```python
from build123d import *

# Parameters (mm, degrees)
F0_W        = 457.2
F0_H        = 88.9
F1_DEPTH    = 12.7
F3_DEPTH    = 12.701
F4_T1_DEPTH = 425.4697854373
F4_T3_DEPTH = 32.2962243683
F4_T5_DEPTH = 24.3646579033


# Not quite as in the source:
# - a fillet or chamfer that OpenCascade refuses, or shapes differently, is made with other operations: its cross-section is extruded or revolved along the edge and cut away or added
# - a feature names something its author has since deleted; it is built from what else it names


with BuildPart() as f1:
    # F0 (on Front) → F1 (new body)
    with BuildSketch(Plane.XZ):
        Rectangle(F0_W, F0_H)
    extrude(amount=F1_DEPTH)

    # F2 (on face) → F3 (cut, through all)
    with BuildSketch(Plane.XZ.offset(12.7)):
        Polygon((-177.273561069, -44.45), (-228.6, 44.45), (-228.6, -44.45), align=None)
    extrude(amount=-F3_DEPTH, mode=Mode.SUBTRACT)

    # F4: chamfer of 3.81 on 4 edges, made by hand

    # F4_s2 → F4_t1 (cut)
    with BuildSketch(Plane.YZ.offset(-187.0716732532)):
        Polygon((0, -40.64), (-3.81, -44.45), (0, -44.45), align=None)
        Polygon((-12.7, -40.64), (-8.89, -44.45), (-12.7, -44.45), align=None)
    extrude(amount=F4_T1_DEPTH, mode=Mode.SUBTRACT)

    # F4_s4 → F4_t3 (cut)
    with BuildSketch(Plane.XZ.offset(-9.7981121842)):
        Polygon((228.6, -40.64), (224.79, -44.45), (228.6, -44.45), align=None)
    extrude(amount=F4_T3_DEPTH, mode=Mode.SUBTRACT)

    # F4_s6 → F4_t5 (cut)
    with BuildSketch(Plane.XZ.offset(-5.8323289516)):
        Polygon((-178.3734133318, -42.545), (-175.0738565434, -44.45), (-177.273561069, -44.45), align=None)
    extrude(amount=F4_T5_DEPTH, mode=Mode.SUBTRACT)


solid = f1.part
```
The listing builds one solid part. Answer for the finished solid, in the listing's coordinates (mm). Round coordinates to 2 decimals unless told otherwise and drop trailing zeros. Order: outer loops, then holes, each group sorted by start corner. A loop starts at its lowest first (then second) coordinate and runs counter-clockwise, first axis right, second up. Notation, with made-up numbers: (-15, 18.25) - (5, 18.25) arc R11 ccw to (5, 37.25) - close; hole circle Ø10 at (6, 1.5). An arc over 180 degrees is marked (long way). Put each result on its own line as item: value. Start each with the question number.
(1) Straight lines are drawn through the part: probe 1 along Z at (x, y) = (-54.5, -12); probe 2 along Z at (x, y) = (127.5, -1); probe 3 along X at (y, z) = (-4, -1). For each, find the intervals that lie inside material, in ascending order. Write a range as from..to.
(2) Given P1, Ø5, axis at y = -3, z = 12, coming from the -X side; P2, Ø1, axis at x = -43, y = -10, coming from the -Z side, each flat-ended and moving along its own axis, determine where each tip first touches the part or whether it passes through.
(3) Find section C-C (z = 21.5). Give the vertices of the cut face in (x, y), plus the area to 3 significant figures.
(4) Find section A-A (y = -6). Give the vertices of the cut face in (x, z) (3 decimals).
(5) Find section B-B (z = -13.5). Give the vertices of the cut face in (x, y), plus the area to 3 significant figures.
Reply:
1. probe 1: -41.34..44.45
1. probe 2: -41.64..44.45
1. probe 3: -202.36..228.6
2. P1: x = -211.31
2. P2: z = -43.84
3. outline: (-215.35, -12.7) - (228.6, -12.7) - (228.6, 0) - (-215.35, 0) - close
3. area: 5,640 mm^2
4. outline: (-228.6, 44.45) - (-178.373, -42.545) - (-175.074, -44.45) - (224.79, -44.45) - (228.6, -40.64) - (228.6, 44.45) - close
5. outline: (-195.14, -12.7) - (228.6, -12.7) - (228.6, 0) - (-195.14, 0) - close
5. area: 5,380 mm^2
